Here's how the part is built. I have some questions about the finished solid (model axes, mm). Give positions to 0.01 mm unless a question says otherwise; leave off trailing zeros. Loops run counter-clockwise (first coordinate to the right, second up) from the corner with the lowest first, then second, coordinate; pieces in that order, holes last. Notation, with made-up numbers: (50.25, 9.5) -> (84.25, 9.5) arc R27 cw to (84.25, 26.5) -> close; hole circle Ø7 at (63, 45). An arc over 180 degrees is marked (long way). Answer in a Markdown table with one row per item. Add a question column.
Item 1: We'd pull the mould along Y, two halves only. Please class faces 1 (the face through (2522, 1947, 0)), 2 (the face through (2496.648, 1985.602, 0.986)), 3 (the face through (2573.99, 1907.38, 0.99)), 4 (the face through (2571.39, 1983.18, 0.99)): released by +Y, released by -Y, zero draft, split by the parting line, or undercut.
Item 2: If I drill on line 1 (X direction, y = 1949.5, z = 0.45); line 2 (X direction, y = 1911, z = 1.75) (3 decimals); line 3 (Y direction, x = 2532, z = 1.1), over which ranges is the centre line in solid material (lowest first)?
Item 3: If we section it at B-B (z = 0.35): Give the number of separate pieces and of enclosed holes in the cut face, then the cut area to 3 significant figures.
Item 4: If we section it at A-A (y = 1965.5): Write out the boundary of the cut face in (x, z).
Item 5: For P1, Ø1, axis at y = 1973.5, z = 1, coming from the +X side; P2, Ø3.5, axis at x = 2570.32, y = 1911.49, coming from the -Z side, each with a flat end and sliding along its axis, tell me the tip position at first contact or that it passes through.
Item 6: If we section it at C-C (y = 1987): Write out the boundary of the cut face in (x, z).
```python
from build123d import *

# Parameters (mm, degrees)
MODEL_R             = 2
EXTRUDE_1_DEPTH     = 2
SKETCH_3_W          = 0.1
SKETCH_3_H          = 8
CUT_EXTRUDE_1_DEPTH = 2
SKETCH_6_W          = 0.1
SKETCH_6_H          = 8
CUT_EXTRUDE_2_DEPTH = 2


with BuildPart() as part:
    # Model → 凸台-拉伸1 (new body)
    with BuildSketch(Plane.XY):
        with BuildLine():
            Line((2557.684762722, 2001.48951402), (2512.949697986, 2001.48951402))
            ThreePointArc((2512.949697986, 2001.48951402), (2512.567014553, 2001.413393553), (2512.242591205, 2001.196620802))
            Line((2512.242591205, 2001.196620802), (2480.610123573, 1969.56415317))
            ThreePointArc((2480.610123573, 1969.56415317), (2480.393350821, 1969.239729821), (2480.317230354, 1968.857046389))
            Line((2480.317230354, 1968.857046389), (2480.317230354, 1924.121981652))
            ThreePointArc((2480.317230354, 1924.121981652), (2480.393350821, 1923.73929822), (2480.610123573, 1923.414874871))
            Line((2480.610123573, 1923.414874871), (2512.242591205, 1891.782407239))
            ThreePointArc((2512.242591205, 1891.782407239), (2512.567014553, 1891.565634488), (2512.949697986, 1891.48951402))
            Line((2512.949697986, 1891.48951402), (2557.684762722, 1891.48951402))
            ThreePointArc((2557.684762722, 1891.48951402), (2558.067446154, 1891.565634488), (2558.391869503, 1891.782407239))
            Line((2558.391869503, 1891.782407239), (2590.024337135, 1923.414874871))
            ThreePointArc((2590.024337135, 1923.414874871), (2590.241109886, 1923.73929822), (2590.317230354, 1924.121981652))
            Line((2590.317230354, 1924.121981652), (2590.317230354, 1968.857046389))
            ThreePointArc((2590.317230354, 1968.857046389), (2590.241109886, 1969.239729821), (2590.024337135, 1969.56415317))
            Line((2590.024337135, 1969.56415317), (2558.391869503, 2001.196620802))
            ThreePointArc((2558.391869503, 2001.196620802), (2558.067446154, 2001.413393553), (2557.684762722, 2001.48951402))
        make_face()
        with Locations((2500.315444685, 1911.487728352)):
            Circle(MODEL_R, mode=Mode.SUBTRACT)
        with Locations((2570.319016023, 1981.491299689)):
            Circle(MODEL_R, mode=Mode.SUBTRACT)
        with Locations((2530.317230354, 1980.496859135)):
            Circle(MODEL_R, mode=Mode.SUBTRACT)
        with Locations((2540.317230354, 1932.196859135)):
            Circle(MODEL_R, mode=Mode.SUBTRACT)
        with Locations((2540.317230354, 1980.496859135)):
            Circle(MODEL_R, mode=Mode.SUBTRACT)
        with Locations((2500.315444685, 1981.491299689)):
            Circle(MODEL_R, mode=Mode.SUBTRACT)
        with Locations((2570.319016023, 1911.487728352)):
            Circle(MODEL_R, mode=Mode.SUBTRACT)
        with Locations((2530.317230354, 1932.196859135)):
            Circle(MODEL_R, mode=Mode.SUBTRACT)
        Polygon((2535.967230354, 1976.491859135), (2535.967230354, 1984.491859135), (2534.667230354, 1984.491859135), (2534.667230354, 1976.491859135), (2525.357779796, 1976.491859135), (2525.357779796, 1936.191859135), (2534.667230354, 1936.191859135), (2534.667230354, 1928.191859135), (2535.967230354, 1928.191859135), (2535.967230354, 1936.191859135), (2545.276680912, 1936.191859135), (2545.276680912, 1976.491859135), align=None, mode=Mode.SUBTRACT)
    extrude(amount=EXTRUDE_1_DEPTH)

    # 草图3 → 切除-拉伸1 (cut)
    with BuildSketch(Plane.XY.offset(2)):
        with Locations((2536.017230354, 1932.191859135)):
            Rectangle(SKETCH_3_W, SKETCH_3_H)
        with Locations((2534.617230354, 1932.191859135)):
            Rectangle(SKETCH_3_W, SKETCH_3_H)
    extrude(amount=-CUT_EXTRUDE_1_DEPTH, mode=Mode.SUBTRACT)

    # 草图6 → 切除-拉伸2 (cut)
    with BuildSketch(Plane.XY.offset(2)):
        with Locations((2536.017230354, 1980.491859135)):
            Rectangle(SKETCH_6_W, SKETCH_6_H)
        with Locations((2534.617230354, 1980.491859135)):
            Rectangle(SKETCH_6_W, SKETCH_6_H)
    extrude(amount=-CUT_EXTRUDE_2_DEPTH, mode=Mode.SUBTRACT)


solid = part.part
```
Recorded:
| question | item | result |
|---|---|---|
| 1 | face 1 | zero draft |
| 1 | face 2 | released by +Y |
| 1 | face 3 | released by -Y |
| 1 | face 4 | undercut |
| 2 | line 1 | x = 2480.32 to 2525.36, 2545.28 to 2590.32 |
| 2 | line 2 | x = 2493.025 to 2498.376, 2502.255 to 2568.379, 2572.259 to 2577.609 |
| 2 | line 3 | y = 1891.49 to 1931.12, 1933.28 to 1936.19, 1976.49 to 1979.42, 1981.58 to 2001.49 |
| 3 | separate pieces | 1 |
| 3 | enclosed holes | 9 |
| 3 | area | 9,100 mm^2 |
| 4 | outline | (2480.32, 0) -> (2525.36, 0) -> (2525.36, 2) -> (2480.32, 2) -> close; (2545.28, 0) -> (2590.32, 0) -> (2590.32, 2) -> (2545.28, 2) -> close |
| 5 | P1 | stops at x = 2586.59 |
| 5 | P2 | passes through |
| 6 | outline | (2498.05, 0) -> (2572.59, 0) -> (2572.59, 2) -> (2498.05, 2) -> close |
